from build123d import *

# Parameters (mm, degrees)
SKETCH1_W               = 34
SKETCH1_H               = 20.5
COMPONENT_OUTLINE_DEPTH = 1
CUT_EXTRUDE1_REACH      = 3
SKETCH4_R               = 0.498272188
SKETCH5_R               = 1.25
CUT_EXTRUDE2_DEPTH      = 2
FILLET1_R               = 2


with BuildPart() as part:
    # Sketch1 → Component_Outline (new body)
    with BuildSketch(Plane.XY):
        with Locations((1.76, 0.09)):
            Rectangle(SKETCH1_W, SKETCH1_H)
    extrude(amount=COMPONENT_OUTLINE_DEPTH)

    # Sketch4 → Cut-Extrude1 (cut, up to next)
    with BuildSketch(Plane.XY.offset(1), mode=Mode.PRIVATE) as cut_extrude1_sk1:
        with Locations((-4.706120495, -7.675571956)):
            Circle(SKETCH4_R)
    cut_extrude1_tool1 = extrude(cut_extrude1_sk1.sketch, amount=-CUT_EXTRUDE1_REACH, mode=Mode.PRIVATE) & part.part
    add(cut_extrude1_tool1.solids().sort_by_distance((-4.70612, -7.675572, 1))[0], mode=Mode.SUBTRACT)
    # Sketch4 → Cut-Extrude1 (cut, up to next)
    with BuildSketch(Plane.XY.offset(1), mode=Mode.PRIVATE) as cut_extrude1_sk2:
        with Locations((-2.166120495, -7.675571956)):
            Circle(SKETCH4_R)
    cut_extrude1_tool2 = extrude(cut_extrude1_sk2.sketch, amount=-CUT_EXTRUDE1_REACH, mode=Mode.PRIVATE) & part.part
    add(cut_extrude1_tool2.solids().sort_by_distance((-2.16612, -7.675572, 1))[0], mode=Mode.SUBTRACT)
    # Sketch4 → Cut-Extrude1 (cut, up to next)
    with BuildSketch(Plane.XY.offset(1), mode=Mode.PRIVATE) as cut_extrude1_sk3:
        with Locations((0.373879505, -7.675571956)):
            Circle(SKETCH4_R)
    cut_extrude1_tool3 = extrude(cut_extrude1_sk3.sketch, amount=-CUT_EXTRUDE1_REACH, mode=Mode.PRIVATE) & part.part
    add(cut_extrude1_tool3.solids().sort_by_distance((0.37388, -7.675572, 1))[0], mode=Mode.SUBTRACT)
    # Sketch4 → Cut-Extrude1 (cut, up to next)
    with BuildSketch(Plane.XY.offset(1), mode=Mode.PRIVATE) as cut_extrude1_sk4:
        with Locations((2.913879505, -7.675571956)):
            Circle(SKETCH4_R)
    cut_extrude1_tool4 = extrude(cut_extrude1_sk4.sketch, amount=-CUT_EXTRUDE1_REACH, mode=Mode.PRIVATE) & part.part
    add(cut_extrude1_tool4.solids().sort_by_distance((2.91388, -7.675572, 1))[0], mode=Mode.SUBTRACT)
    # Sketch4 → Cut-Extrude1 (cut, up to next)
    with BuildSketch(Plane.XY.offset(1), mode=Mode.PRIVATE) as cut_extrude1_sk5:
        with Locations((5.453879505, -7.675571956)):
            Circle(SKETCH4_R)
    cut_extrude1_tool5 = extrude(cut_extrude1_sk5.sketch, amount=-CUT_EXTRUDE1_REACH, mode=Mode.PRIVATE) & part.part
    add(cut_extrude1_tool5.solids().sort_by_distance((5.45388, -7.675572, 1))[0], mode=Mode.SUBTRACT)
    # Sketch4 → Cut-Extrude1 (cut, up to next)
    with BuildSketch(Plane.XY.offset(1), mode=Mode.PRIVATE) as cut_extrude1_sk6:
        with Locations((7.993879505, -7.675571956)):
            Circle(SKETCH4_R)
    cut_extrude1_tool6 = extrude(cut_extrude1_sk6.sketch, amount=-CUT_EXTRUDE1_REACH, mode=Mode.PRIVATE) & part.part
    add(cut_extrude1_tool6.solids().sort_by_distance((7.99388, -7.675572, 1))[0], mode=Mode.SUBTRACT)

    # Sketch5 → Cut-Extrude2 (cut, through all)
    with BuildSketch(Plane.XY.offset(1)):
        with Locations((-13.24, 8.34)):
            Circle(SKETCH5_R)
        with Locations((16.76, 8.34)):
            Circle(SKETCH5_R)
        with Locations((16.76, -8.16)):
            Circle(SKETCH5_R)
        with Locations((-13.24, -8.16)):
            Circle(SKETCH5_R)
    extrude(amount=-CUT_EXTRUDE2_DEPTH, mode=Mode.SUBTRACT)

    # Fillet1
    fillet1_edges = [part.edges().sort_by_distance(p)[0] for p in [
        (-15.24, 10.34, 0.5),
        (18.76, 10.34, 0.5),
        (18.76, -10.16, 0.5),
        (-15.24, -10.16, 0.5),
    ]]
    fillet(fillet1_edges, radius=FILLET1_R)


solid = part.part
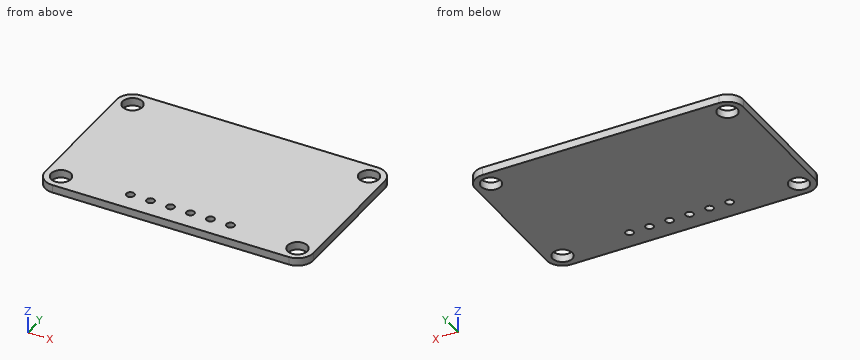
Geometry check sheet. Reference: the model listing, model coordinates, mm. Round coordinates to 2 decimals unless told otherwise and drop trailing zeros. One line per item, written item: value. Start each with the question number.
(1) Scan line: line 1 (X direction, y = 9.25, z = 0.95). Record every from-to range of solid material in increasing order. Write a range as [from, to].
(2) Go/stop test with a flat-tipped pin: pin 1 Ø2 at (x, y) = (16.76, 8.34) entering from +Z. Record where the tip stops, or that it passes through.
(3) Cross-section at A-A, the plane z = 0.65. Give the number of separate pieces and of enclosed holes in the cut face, and give its area (3 significant figures).
Answer:
1. line 1: [-15.02, -14.1], [-12.38, 15.9], [17.62, 18.54]
2. pin 1: through
3. separate pieces: 1
3. enclosed holes: 10
3. area: 669 mm²
